Here's the drawing with two shaded views (mm, measured from the low corner). I have some questions. A direction names the side the tool comes from. Round coordinates to 2 decimals unless told otherwise and drop trailing zeros. Order: outer loops, then holes, each group sorted by start corner. A loop starts at its lowest first (then second) coordinate and runs counter-clockwise, first axis right, second up. Notation, with made-up numbers: (16.25, -10.5) -> (72.25, -10.5) arc R22 ccw to (72.25, 6.5) -> close; hole circle Ø6 at (26, 5.5). An arc over 180 degrees is marked (long way). Answer in a Markdown table with one row per item.
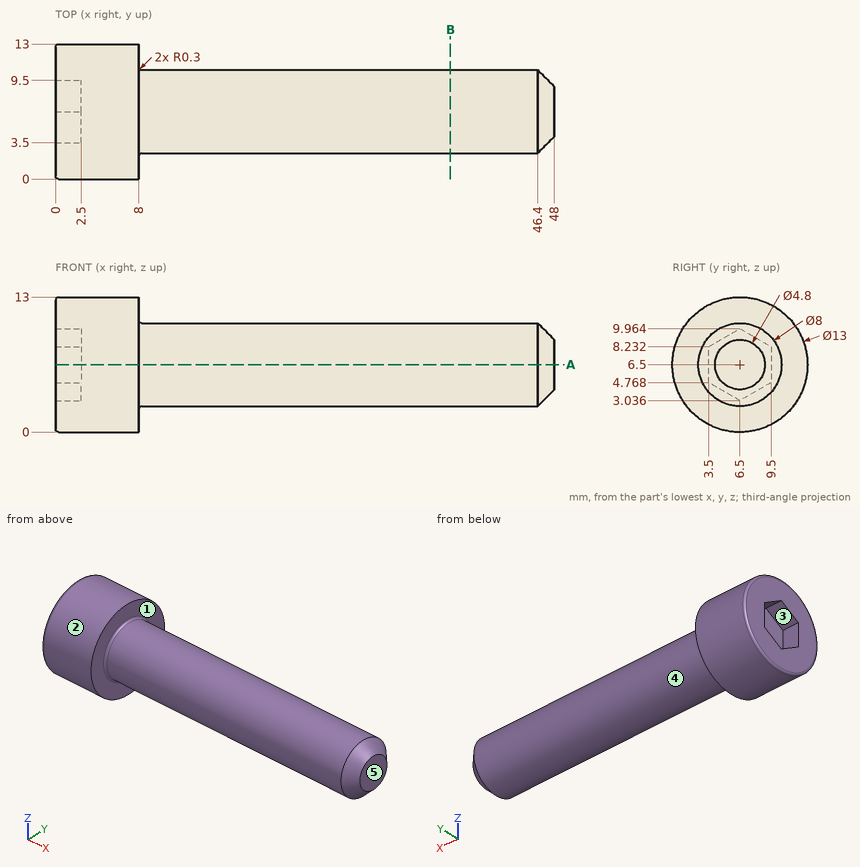
1. Suppose I cut it at A-A on z = 6.5. Write out the boundary of the cut face in (x, y), then the cut area to 3 significant figures.
Numbers:
| item | result |
|---|---|
| outline | (0, 0.3) arc R0.3 ccw to (0.3, 0) -> (8, 0) -> (8, 2.2) arc R0.3 cw to (8.3, 2.5) -> (46.4, 2.5) -> (48, 4.1) -> (48, 8.9) -> (46.4, 10.5) -> (8.3, 10.5) arc R0.3 cw to (8, 10.8) -> (8, 13) -> (0.3, 13) arc R0.3 ccw to (0, 12.7) -> (0, 9.5) -> (2.5, 9.5) -> (2.5, 3.5) -> (0, 3.5) -> close |
| area | 406 mm2 |
2. We'd pull the mould along Z, two halves only. Please class the marked faces 3, 4 and 5: released by +Z, released by -Z, zero draft, split by the parting line, or undercut.
Numbers:
| item | result |
|---|---|
| face 3 | undercut |
| face 4 | split by the parting line |
| face 5 | zero draft |
3. Please list where these lines run through material, in increasing order: line 1 along X through (y, z) = (2.25, 2.25); line 2 along Z through (x, y) = (36, 6.75); line 3 along X through (y, z) = (6, 4.5).
Numbers:
| item | result |
|---|---|
| line 1 | x = 0 to 8 |
| line 2 | z = 2.51 to 10.49 |
| line 3 | x = 2.5 to 48 |
4. For pin 1 Ø1 at (x, y) = (34.5, 5) entering from +Z; pin 2 Ø1.5 at (x, y) = (43, 6.5) entering from +Z; pin 3 Ø2 at (y, z) = (3, 6.5) entering from +X, each with a flat end and sliding along its axis, tell me the tip position at first contact or that it passes through.
Numbers:
| item | result |
|---|---|
| pin 1 | stops at z = 10.37 |
| pin 2 | stops at z = 10.5 |
| pin 3 | stops at x = 47.9 |
5. For the marked faces 1 and 2, which set-ups out of +Z, -Z, +X, -X, +Y, -Y let a thin tool reach every point of the face, with its end or its side?
Numbers:
| item | result |
|---|---|
| face 1 | +X |
| face 2 | +X, -X |
6. Suppose I cut it at B-B on x = 38. Write out the boundary of the cut face in (y, z), then the cut area to 3 significant figures.
Numbers:
| item | result |
|---|---|
| outline | circle Ø8 at (6.5, 6.5) |
| area | 50.3 mm2 |
